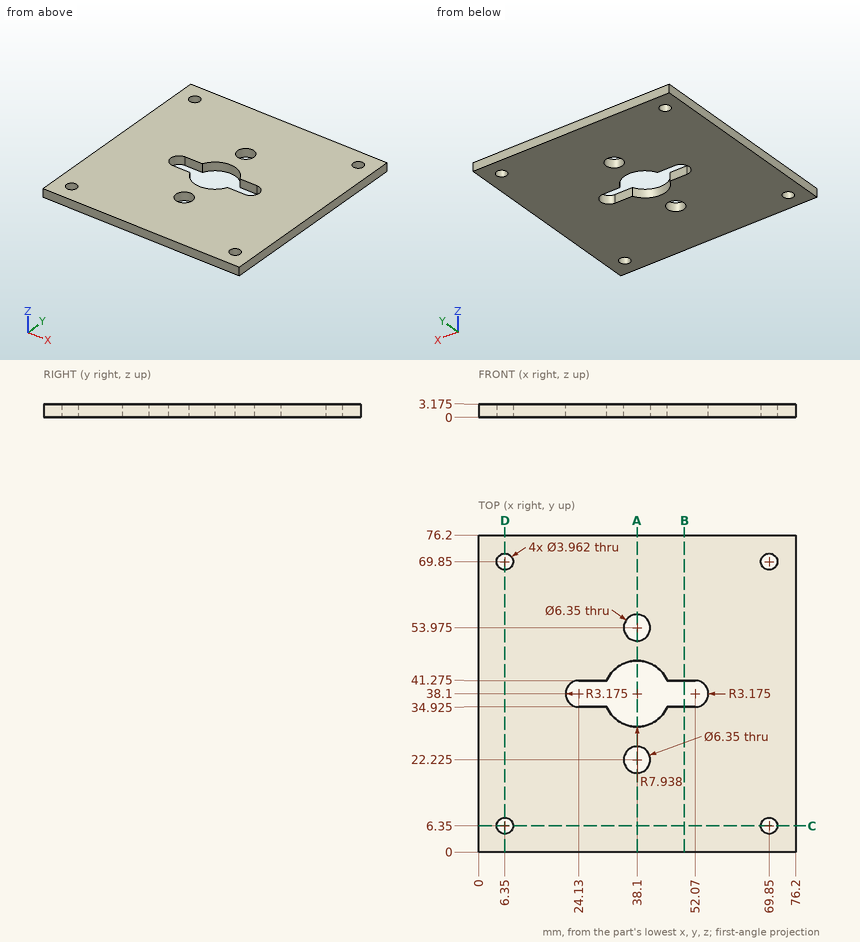
Part print with two shaded views. Sizes in mm from the minimum x, y, z corner. Coordinates: 2 decimals unless noted, no trailing zeros. Write each loop counter-clockwise with the first axis right and the second up, starting at its lowest first coordinate (ties: lowest second). Pieces come first, ordered by that corner, then holes.
(1) Cut at A-A on x = 38.1. State how many separate pieces and enclosed holes the cut face has, and give its area (3 significant figures).
(2) Cut at B-B on x = 49.5. List the corners of the cut face in (y, z) (1 decimal).
(3) Pin check, flat tip, straight feed: pin 1 Ø2.5 at (x, y) = (6.35, 69.85) entering from +Z. Stop position of the tip, or through.
(4) Drill centre lines: line 1 (X direction, y = 6.35, z = 2.4); line 2 (Y direction, x = 38.1, z = 1.65). Where is each one in solid material? Low to high.
(5) Cut at C-C on y = 6.35. List the corners of the cut face in (x, z) (1 decimal), and give its area (3 significant figures).
Working result:
1. separate pieces: 4
1. enclosed holes: 0
1. area: 151 mm2
2. outline: (0, 0) - (34.9, 0) - (34.9, 3.2) - (0, 3.2) - close; (41.3, 0) - (76.2, 0) - (76.2, 3.2) - (41.3, 3.2) - close
3. pin 1: passes through
4. line 1: x = 0 to 4.37, 8.33 to 67.87, 71.83 to 76.2
4. line 2: y = 0 to 19.05, 25.4 to 30.16, 46.04 to 50.8, 57.15 to 76.2
5. outline: (0, 0) - (4.4, 0) - (4.4, 3.2) - (0, 3.2) - close; (8.3, 0) - (67.9, 0) - (67.9, 3.2) - (8.3, 3.2) - close; (71.8, 0) - (76.2, 0) - (76.2, 3.2) - (71.8, 3.2) - close
5. area: 217 mm2
